```python
from build123d import *

# Parameters (mm, degrees)
CHAMFER1_SIZE = 0.25


with BuildPart() as part:
    # Sketch2 → Revolve1 (revolve)
    with BuildSketch(Plane(origin=(0, 0, 0), x_dir=(1, 0, 0), z_dir=(0, 1, 0))):
        Polygon((-4.762498993, -2.9131e-05), (-11.112498283, -2.9131e-05), (-11.112498283, -5.638830007), (-12.344399539, -5.638830007), (-12.344399539, -7.162829152), (-4.762498993, -7.162829152), align=None)
    revolve(axis=Axis((0, 0, 0), (0, 0, 1)))

    # Chamfer1
    chamfer1_edges = [part.edges().sort_by_distance(p)[0] for p in [
        (11.112498283, 0, 2.9131e-05),
        (4.762498993, 0, 2.9131e-05),
        (4.762498993, 0, 7.162829152),
        (12.344399539, 0, 7.162829152),
        (12.344399539, 0, 5.638830007),
    ]]
    chamfer(chamfer1_edges, length=CHAMFER1_SIZE)


solid = part.part
```
For this review, take the finished solid that the model builds, in its own axes (mm). Coordinates: 2 decimals unless noted, no trailing zeros. Loops run counter-clockwise (first coordinate to the right, second up) from the corner with the lowest first, then second, coordinate; pieces in that order, holes last.
1. Add section C-C, the plane z = 4. Give the boundary of the cut face in (x, y) (1 decimal), then the cut area to 3 significant figures.
2. For line 1 (Y direction, x = 0, z = 5.5); line 2 (X direction, y = 4, z = 6.5), list the stretches that pass through material, from the lowest coordinate up.
3. Add section A-A, the plane y = 0. Give the boundary of the cut face in (x, z), then the cut area to 3 significant figures.
4. Mouldability with a two-part tool opening along Y and no side actions: class faces 1 (the cylindrical face through (8.82, 6.76, 2.98)), 2 (the flat face through (11, 4, 5.639)), 3 (the cylindrical face through (0.62, -4.72, 3.53)) as +Y half, -Y half, draft (parallel to the pull), parting line (faces both ways), or undercut.
5. Insertion check: P1, Ø4, axis at y = -7.5, z = 5.5, coming from the -X side; P2, Ø2, axis at y = -4.5, z = 2, coming from the +X side; P3, Ø8.5, axis at x = 0, y = 0, coming from the -Z side. Each pin has a flat end and moves straight along its axis. Give the tip position at first contact, or say it passes through.
Result:
1. outline: circle Ø22.2 at (0, 0); hole circle Ø9.5 at (0, 0)
1. area: 317 mm2
2. line 1: y = -11.11 to -4.76, 4.76 to 11.11
2. line 2: x = -11.68 to -2.58, 2.58 to 11.68
3. outline: (-12.34, 5.89) - (-12.09, 5.64) - (-11.11, 5.64) - (-11.11, 0.25) - (-10.86, 0) - (-5.01, 0) - (-4.76, 0.25) - (-4.76, 6.91) - (-5.01, 7.16) - (-12.09, 7.16) - (-12.34, 6.91) - close; (4.76, 0.25) - (5.01, 0) - (10.86, 0) - (11.11, 0.25) - (11.11, 5.64) - (12.09, 5.64) - (12.34, 5.89) - (12.34, 6.91) - (12.09, 7.16) - (5.01, 7.16) - (4.76, 6.91) - close
3. area: 94.4 mm2
4. face 1: parting line
4. face 2: draft
4. face 3: undercut
5. P1: stops at x = -11.03
5. P2: stops at x = 10.55
5. P3: passes through
